Part model, mm, in its own coordinate system. A direction names the side the tool comes from. Coordinates: 2 decimals unless noted, no trailing zeros. Loops run counter-clockwise (first coordinate to the right, second up) from the corner with the lowest first, then second, coordinate; pieces in that order, holes last. Notation, with made-up numbers: M 8,-10.5 L 61,-10.5 A23 cw 61,3.5 Z; hole C -35,86.25 d10. An arc over 180 degrees is marked long. Use a Markdown table: item, result. Add a question column.
1) Pull direction Z, two halves, no side cores. Call faces 3 (the flat face through (2, 69, 0)), 4 (the flat face through (0, 69, -79)), 5 (the flat face through (2, 3, -110)): released by +Z, released by -Z, zero draft, split by the parting line, or undercut.
2) Wall check: probe 1 along Y at (x, z) = (4.7, -66.5); probe 2 along Y at (x, z) = (3.7, -64.5); probe 3 along Z at (x, y) = (2.45, 21). Give the ranges that are in metal, low to high. Write a range as from..to.
3) Tool access for faces 1 (the flat face through (2, 140, -79)), 2 (the flat face through (2, 5, -80)): list every direction of +Z, -Z, +X, -X, +Y, -Y with a clear straight run to the whole face (end or side of a thin tool).
4) Band-saw the part on A-A (z = -76.5). List the corners of the cut face in (x, y).
5) Pin check, flat tips, straight feed: pin 1 Ø2.5 at (x, z) = (1.5, -68.5) entering from -Y; pin 2 Ø2.5 at (y, z) = (121.53, -92.95) entering from +X. Stop position of each tip, or through.
Autodesk Inventor part; units mm, degrees
ref_plane "YZ Plane" through (0, 0, 0) normal (1, 0, 0) x (0, 1, 0)
ref_plane "XZ Plane" through (0, 0, 0) normal (0, 1, 0) x (-1, 0, 0)
ref_plane "XY Plane" through (0, 0, 0) normal (0, 0, 1) x (1, 0, 0)
sketch "Sketch1" plane through (0, 0, 0) normal (1, 0, 0) x (0, 1, 0)
  line L0 (0, 0) -> (140, 0)
  line L1 (140, 0) -> (140, -160)
  line L2 (140, -160) -> (0, -160)
  line L3 (0, -160) -> (0, 0)
  line L4 (0, -50) -> (5, -50)
  line L5 (5, -50) -> (5, -110)
  line L6 (5, -110) -> (0, -110)
  line L7 (0, -110) -> (0, -50)
  point P0 (0, -110)
  dimension "d0" = 140
  dimension "d1" = 160
  dimension "d2" = 5
  dimension "d3" = 60
  dimension "d4" = 50
extrude "Extrusion1" add sketch "Sketch1" along normal blind 5 contours L0 L1 L2 L3 L6 L5 L4
sketch "Sketch2" plane through (5, 0, 0) normal (1, 0, 0) x (0, 0, -1)
  line L0 (0, 0) -> (50, 0)
  line L1 (50, 0) -> (50, 5)
  point P0 (80, 20)
  dimension "d14" = 20
  dimension "d15" = 30
hole "Hole1" at (5, 20, -80) direction (-1, 0, 0) diameter 3 end through all
sketch "Sketch12" plane through (5, 0, 0) normal (1, 0, 0) x (0, 0, -1)
  circle A0 centre (95.2983, 42.3183) radius 1.5
  circle A1 centre (92.9456, 121.5257) radius 1.5
  circle A2 centre (70.9676, 122.7958) radius 1.5
  circle A3 centre (66.5863, 42.8118) radius 1.5
  point P0 (0, 0)
extrude "Extrusion5" cut sketch "Sketch12" against normal through all
properties part number "TOP_1"
Entries:
| question | item | result |
|---|---|---|
| 1 | face 3 | released by +Z |
| 1 | face 4 | zero draft |
| 1 | face 5 | undercut |
| 2 | probe 1 | 5..41.31, 44.31..140 |
| 2 | probe 2 | 5..140 |
| 2 | probe 3 | -160..-81.12, -78.88..0 |
| 3 | face 1 | +Z, -Z, +X, -X, +Y |
| 3 | face 2 | +X, -X, -Y |
| 4 | outline | M 0,5 L 5,5 L 5,140 L 0,140 Z |
| 5 | pin 1 | y = 5 |
| 5 | pin 2 | through |
